For this review, take the finished solid that the model builds, in its own axes (mm). Give positions to 0.01 mm unless a question says otherwise; leave off trailing zeros. Order: outer loops, then holes, each group sorted by start corner. A loop starts at its lowest first (then second) coordinate and runs counter-clockwise, first axis right, second up.
Autodesk Inventor part; units mm, degrees
ref_plane "YZ Plane" through (0, 0, 0) normal (1, 0, 0) x (0, 1, 0)
ref_plane "XZ Plane" through (0, 0, 0) normal (0, 1, 0) x (-1, 0, 0)
ref_plane "XY Plane" through (0, 0, 0) normal (0, 0, 1) x (1, 0, 0)
sketch "Sketch1" plane through (0, 0, 0) normal (0, 0, 1) x (1, 0, 0)
  line L0 (0, 0) -> (381, 0)
  line L1 (381, 0) -> (381, 50.8)
  line L2 (381, 50.8) -> (0, 50.8)
  line L3 (0, 50.8) -> (0, 0)
  circle A0 centre (12.7, 12.7) radius 2.0701
  circle A1 centre (12.7, 38.1) radius 2.0701
  circle A2 centre (368.3, 12.7) radius 2.0701
  circle A3 centre (368.3, 38.1) radius 2.0701
  dimension "d0" = 50.8
  dimension "d1" = 381
  dimension "d2" = 4.1402
  dimension "d3" = 12.7
  dimension "d4" = 12.7
  dimension "d7" = 25.4
  dimension "d10" = 355.6
extrude "Extrusion1" add sketch "Sketch1" along normal blind 3.175
sketch "Sketch2" plane through (0, 0, 3.175) normal (0, 0, 1) x (1, 0, 0)
  line L0 (0, 0) -> (381, 0)
  line L1 (0, 50.8) -> (0, 0)
  line L2 (152.4, 0) -> (114.3, 0)
  line L3 (114.3, 0) -> (114.3, 31.75)
  line L4 (114.3, 31.75) -> (152.4, 31.75)
  line L5 (152.4, 31.75) -> (152.4, 0)
  dimension "d15" = 31.75
  dimension "d16" = 38.1
  dimension "d17" = 114.3
extrude "Extrusion2" cut sketch "Sketch2" against normal blind 25.4
properties part number "Polycarbonate Sheet" material "Polycarbonate, Clear"
1) We need section A-A on y = 24.5. Give the boundary of the cut face in (x, z) (3 decimals), then the cut area to 3 significant figures.
Answer sheet:
outline: (0, 0) - (114.3, 0) - (114.3, 3.175) - (0, 3.175) - close; (152.4, 0) - (381, 0) - (381, 3.175) - (152.4, 3.175) - close
area: 1,090 mm2
2) We need section B-B on z = 2.4. Give the boundary of the cut face in (x, y), then the cut area to 3 significant figures.
Answer sheet:
outline: (0, 0) - (114.3, 0) - (114.3, 31.75) - (152.4, 31.75) - (152.4, 0) - (381, 0) - (381, 50.8) - (0, 50.8) - close; hole circle Ø4.14 at (12.7, 12.7); hole circle Ø4.14 at (12.7, 38.1); hole circle Ø4.14 at (368.3, 12.7); hole circle Ø4.14 at (368.3, 38.1)
area: 18,100 mm2
3) To check wall thickness, follow line 1 (Y direction, x = 12.7, z = 1.5); line 2 (X direction, y = 21.5, z = 0.75); line 3 (X direction, y = 14.5, z = 1.95). State the ranges of each line that lie inside material, in increasing order.
Answer sheet:
line 1: y = 0 to 10.63, 14.77 to 36.03, 40.17 to 50.8
line 2: x = 0 to 114.3, 152.4 to 381
line 3: x = 0 to 11.68, 13.72 to 114.3, 152.4 to 367.28, 369.32 to 381
4) We need section C-C on x = 124. Give the boundary of the cut face in (y, z) (3 decimals).
Answer sheet:
outline: (31.75, 0) - (50.8, 0) - (50.8, 3.175) - (31.75, 3.175) - close
5) Clearance check with a flat-ended pin moving along its axis: pin 1 (6.5 mm diameter, centred on x = 12.7, y = 38.1, fed in from -Z). State where the tip first meets the part, or that it passes through.
Answer sheet:
pin 1: stops at z = 0
